Model file for the job. Use its own axes, mm. Round coordinates to 2 decimals unless told otherwise and drop trailing zeros. Order: outer loops, then holes, each group sorted by start corner. A loop starts at its lowest first (then second) coordinate and runs counter-clockwise, first axis right, second up. Notation, with made-up numbers: (77.5, 61.25) - (109.5, 61.25) arc R16 cw to (109.5, 87.25) - close; hole circle Ø6 at (-12, -12.75). An arc over 180 degrees is marked (long way). Answer as CSV lines item,"result". Start each with the question number.
1. Pull direction X, two halves, no side cores. Call faces 1 (the face through (200, 10, 2)), 2 (the face through (99, 20, 2)), 3 (the face through (0, 10, 2)), 4 (the face through (134.77, 11.5, 2.46)): released by +X, released by -X, zero draft, split by the parting line, or undercut.
2. Wall check: line 1 along Y through (x, z) = (190, 1.75); line 2 along Y through (x, z) = (169, 1.1). Give the ranges that are in metal, low to high. Write a range as [from, to].
3. Band-saw the part on A-A on x = 130. List the corners of the cut face in (y, z), then the cut area to 3 significant figures.
4. Pin check, flat tip, straight feed: pin 1 Ø8 at (x, y) = (30, 10) entering from +Z. Stop position of the tip, or through.
5. Band-saw the part on B-B on z = 2.45. State how many separate pieces and enclosed holes the cut face has, then the cut area to 3 significant figures.
```python
from build123d import *

# Parameters (mm, degrees)
SZKIC2_W                    = 200
SZKIC2_H                    = 20
SZKIC2_R                    = 5
DODANIE_WYCI_GNI_CIE5_DEPTH = 5
SZYK_LINIOWY1_OUTLINE_R     = 5
SZYK_LINIOWY1_DEPTH         = 5


# Read off the part's stored shape, not the designer's step: Szyk liniowy1
with BuildPart() as part:
    # Szkic2 → Dodanie-wyciągnięcie5 (new body)
    with BuildSketch(Plane.XY):
        with Locations((100, 10)):
            Rectangle(SZKIC2_W, SZKIC2_H)
        with Locations((10, 10)):
            Circle(SZKIC2_R, mode=Mode.SUBTRACT)
    extrude(amount=DODANIE_WYCI_GNI_CIE5_DEPTH)

    # Szyk liniowy1 outline → Szyk liniowy1 (cut)
    with BuildSketch(Plane.XY):
        with Locations((190, 10)):
            Circle(SZYK_LINIOWY1_OUTLINE_R)
        with Locations((170, 10)):
            Circle(SZYK_LINIOWY1_OUTLINE_R)
        with Locations((150, 10)):
            Circle(SZYK_LINIOWY1_OUTLINE_R)
        with Locations((130, 10)):
            Circle(SZYK_LINIOWY1_OUTLINE_R)
        with Locations((110, 10)):
            Circle(SZYK_LINIOWY1_OUTLINE_R)
        with Locations((90, 10)):
            Circle(SZYK_LINIOWY1_OUTLINE_R)
        with Locations((70, 10)):
            Circle(SZYK_LINIOWY1_OUTLINE_R)
        with Locations((50, 10)):
            Circle(SZYK_LINIOWY1_OUTLINE_R)
        with Locations((30, 10)):
            Circle(SZYK_LINIOWY1_OUTLINE_R)
    extrude(amount=SZYK_LINIOWY1_DEPTH, mode=Mode.SUBTRACT)


solid = part.part
```
Reply:
1,face 1,"released by +X"
1,face 2,"zero draft"
1,face 3,"released by -X"
1,face 4,"undercut"
2,line 1,"y = [0, 5], [15, 20]"
2,line 2,"y = [0, 5.1], [14.9, 20]"
3,outline,"(0, 0) - (5, 0) - (5, 5) - (0, 5) - close; (15, 0) - (20, 0) - (20, 5) - (15, 5) - close"
3,area,"50.0 mm2"
4,pin 1,"passes through"
5,separate pieces,"1"
5,enclosed holes,"10"
5,area,"3,210 mm2"
